from build123d import *

# Parameters (mm, degrees)
F0_W      = 38.1
F0_H      = 31.75
F1_DEPTH  = 44.45
F2_W      = 12.7
F2_H      = 31.75
F3_DEPTH  = 19.05
F5_DEPTH  = 12.7
F7_DEPTH  = 12.7
F8_DEPTH  = 6.35
F10_DEPTH = 25.4


# Not quite as in the source:
# - a feature names something its author has since deleted; it is built from what else it names


with BuildPart() as f1:
    # F0 (on Front) → F1 (new body)
    with BuildSketch(Plane.XZ):
        with Locations((19.05, 15.875)):
            Rectangle(F0_W, F0_H)
    extrude(amount=F1_DEPTH)

    # F2 (on face) → F3 (cut)
    with BuildSketch(Plane.XZ.offset(44.45)):
        with Locations((31.75, 15.875)):
            Rectangle(F2_W, F2_H)
        with Locations((6.35, 15.875)):
            Rectangle(F2_W, F2_H)
    extrude(amount=-F3_DEPTH, mode=Mode.SUBTRACT)

    # F4 (on face) → F5 (cut)
    with BuildSketch(Plane.YZ.offset(38.1)):
        Polygon((-25.4, 0), (-19.05, 31.75), (-25.4, 31.75), align=None)
    extrude(amount=-F5_DEPTH, mode=Mode.SUBTRACT)

    # F6 (on face) → F7 (cut)
    with BuildSketch(Plane(origin=(0, 0, 0), x_dir=(0, -1, 0), z_dir=(-1, 0, 0))):
        Polygon((25.4, 0), (25.4, 31.75), (19.05, 31.75), align=None)
    extrude(amount=-F7_DEPTH, mode=Mode.SUBTRACT)

    # F8 (add): a face of the model
    f8_faces = [f1.faces().sort_by_distance(p)[0] for p in [
        (19.05, -44.45, 15.875),
    ]]
    extrude(f8_faces, amount=F8_DEPTH)

    # F9 (on face) → F10 (cut)
    with BuildSketch(Plane.YZ.offset(25.4)):
        Polygon((-50.8, 0), (-44.45, 31.75), (-50.8, 31.75), align=None)
    extrude(amount=-F10_DEPTH, mode=Mode.SUBTRACT)


solid = f1.part
Check sheet for the modelled part. Datum: model origin and axes. Units: mm. A direction names the side the tool comes from. Round coordinates to 2 decimals unless told otherwise and drop trailing zeros. Order: outer loops, then holes, each group sorted by start corner. A loop starts at its lowest first (then second) coordinate and runs counter-clockwise, first axis right, second up. Notation, with made-up numbers: M -9.75,43.5 L 15.25,43.5 A20 cw 15.25,82.5 Z; hole C 62.25,-25 d6. An arc over 180 degrees is marked long. One line per item, written item: value. Start each with the question number.
1. Section check A-A on z = 16.5. Enter the section's corners in (x, y).
2. Gauge pin test, flat ends, axial feed: P1, Ø12, axis at y = -34.5, z = 13.5, coming from the -X side; P2, Ø1, axis at x = 18, z = 14.5, coming from the -Y side; P3, Ø4, axis at x = 13, z = 15.5, coming from the -Y side. Record the tip position at first contact, or that the pin passes through.
3. Section check B-B on y = -37. Enter the section's corners in (x, z), and give its area (3 significant figures).
4. Access from +Z, -Z, +X, -X, +Y, -Y to the whole of each face (thin tool, end or side, straight path). Record for faces 1 (the flat face through (6.26, -22.18, 16.1)), 2 (the flat face through (25.4, -35, 16)), 3 (the flat face through (19, 0, 16)).
5. Scan lines: line 1 along X through (y, z) = (-47, 7); line 2 along Y through (x, z) = (15.5, 13); line 3 along Y through (x, z) = (4.5, 20.5). Record each from-to range of solid material in increasing order.
6. Section check C-C on x = 15. Enter the section's corners in (y, z), and give its area (3 significant figures).
7. Section check D-D on z = 10. Enter the section's corners in (x, y).
Results found:
1. outline: M 0,-22.1 L 12.7,-22.1 L 12.7,-47.5 L 25.4,-47.5 L 25.4,-22.1 L 38.1,-22.1 L 38.1,0 L 0,0 Z
2. P1: x = 12.7
2. P2: y = -48
2. P3: y = -48.1
3. outline: M 12.7,0 L 25.4,0 L 25.4,31.75 L 12.7,31.75 Z
3. area: 403 mm^2
4. face 1: +Z, -X, -Y
4. face 2: +Z, +X, -Y
4. face 3: +Z, -Z, +X, -X, +Y
5. line 1: 12.7 to 25.4
5. line 2: -48.2 to 0
5. line 3: -21.3 to 0
6. outline: M -50.8,0 L 0,0 L 0,31.75 L -44.45,31.75 Z
6. area: 1,510 mm^2
7. outline: M 0,-23.4 L 12.7,-23.4 L 12.7,-48.8 L 25.4,-48.8 L 25.4,-23.4 L 38.1,-23.4 L 38.1,0 L 0,0 Z
